Check sheet for the drawn part. Datum: minimum x, y, z corner. Units: mm. A direction names the side the tool comes from. Round coordinates to 2 decimals unless told otherwise and drop trailing zeros. Write each loop counter-clockwise with the first axis right and the second up, starting at its lowest first coordinate (ties: lowest second). Pieces come first, ordered by that corner, then holes. Notation, with made-up numbers: M 2.25,-23 L 57.25,-23 A14 ccw 57.25,1 Z; hole C 52.25,-26.75 d7. An arc over 180 degrees is marked long. One line per item, written item: value.
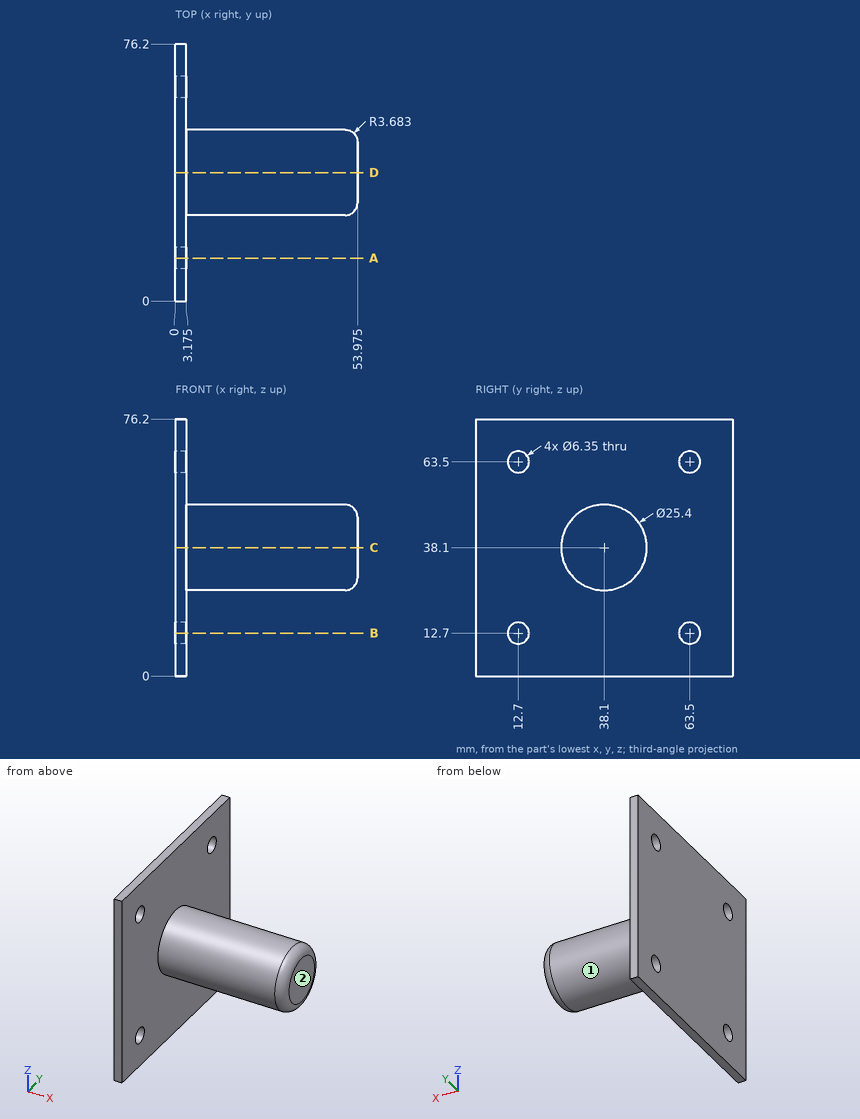
Q1. Sectioned sample at A-A on y = 12.7. Enter the section's corners in (x, z) (1 decimal).
Completed:
outline: M 0,0 L 3.2,0 L 3.2,9.5 L 0,9.5 Z; M 0,15.9 L 3.2,15.9 L 3.2,60.3 L 0,60.3 Z; M 0,66.7 L 3.2,66.7 L 3.2,76.2 L 0,76.2 Z
Q2. Sectioned sample at C-C on z = 38.1. Enter the section's corners in (x, y) (1 decimal), and give its area (3 significant figures).
Completed:
outline: M 0,0 L 3.2,0 L 3.2,25.4 L 50.3,25.4 A3.7 ccw 54,29.1 L 54,47.1 A3.7 ccw 50.3,50.8 L 3.2,50.8 L 3.2,76.2 L 0,76.2 Z
area: 1,530 mm^2
Q3. Access from +Z, -Z, +X, -X, +Y, -Y to the whole of each face (thin tool, end or side, straight path). Record for the marked faces 1 and 2.
Completed:
face 1: +X
face 2: +Z, -Z, +X, +Y, -Y
Q4. Scan lines: line 1 (Y direction, x = 2.15, z = 63.5) (1 decimal); line 2 (X direction, y = 62, z = 58) (1 decimal); line 3 (Y direction, x = 19, z = 28). Record each from-to range of solid material in increasing order. Write a range as [from, to].
Completed:
line 1: [0, 9.5], [15.9, 60.3], [66.7, 76.2]
line 2: [0, 3.2]
line 3: [30.4, 45.8]
Q5. Depth check by flat-ended pin: P1, Ø1.5, axis at x = 28.5, y = 39.5, coming from the -Z side; P2, Ø10, axis at y = 63.5, z = 12.7, coming from the +X side (3 decimals); P3, Ø2, axis at x = 36, z = 23.5, coming from the +Y side; P4, Ø6, axis at x = 28, z = 52.5, coming from the +Y side. Enter the tip coordinate at first touch or a pass-through.
Completed:
P1: z = 25.42
P2: x = 3.175
P3: through
P4: y = 43.7
